The listing builds one solid part. Answer for the finished solid, in the listing's coordinates (mm). Give positions to 0.01 mm unless a question says otherwise; leave off trailing zeros. Loops run counter-clockwise (first coordinate to the right, second up) from the corner with the lowest first, then second, coordinate; pieces in that order, holes last. Notation, with made-up numbers: (-5.75, 38) - (-0.75, 38) arc R28 ccw to (-0.75, 58) - close; hole circle Ø10 at (-30.5, -27.5). An arc over 180 degrees is marked (long way). Answer as CSV lines item,"result". Start each with the question number.
1) A cutting plane is placed at A-A (x = -32.5). Determine the outline of the cut face in (y, z), and give its area (3 significant figures).
2) Flat-ended cylindrical pins translate along their axes: pin 1 (8 mm diameter, centred on x = 179, y = 432.5, fed in from +Z); pin 2 (3.5 mm diameter, centred on x = -203.2, y = 0, fed in from +Z). Find the tip coordinate at first contact, or state that the pin passes through.
3) A cutting plane is placed at C-C (z = 2). Determine the outline of the cut face in (x, y) (3 decimals), and give its area (3 significant figures).
4) A cutting plane is placed at B-B (y = -341). Determine the outline of the cut face in (x, z).
5) Find the intervals of material crossed by line 1 along Y through (x, z) = (-203.2, 5.5); line 2 along X through (y, z) = (787.4, 6.75); line 3 along X through (y, z) = (446, 3.75), in increasing order.
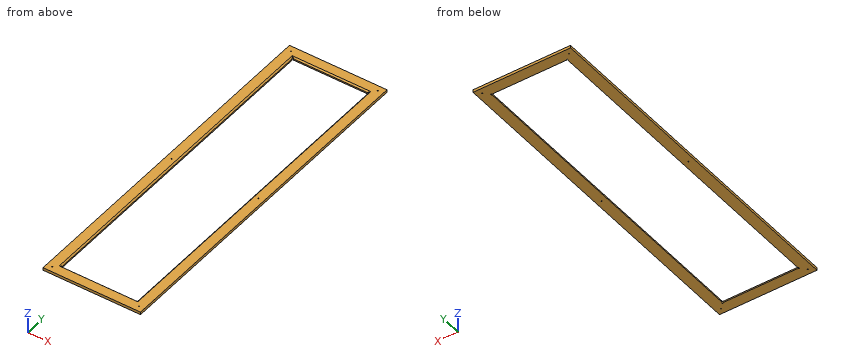
```python
from build123d import *

# Parameters (mm, degrees)
F0_W     = 457.2
F0_H     = 1625.6
F0_W_2   = 355.6
F0_H_2   = 1524
F1_DEPTH = 12.7
F2_SIZE  = 6.35
F3_R     = 3.175
F4_DEPTH = 12.7
F5_R     = 2.15265
F6_DEPTH = 12.7


with BuildPart() as f1:
    # F0 (on Top) → F1 (new body)
    with BuildSketch(Plane.XY):
        Rectangle(F0_W, F0_H)
        Rectangle(F0_W_2, F0_H_2, mode=Mode.SUBTRACT)
    extrude(amount=F1_DEPTH)

    # F2
    f2_edges = [f1.edges().sort_by_distance(p)[0] for p in [
        (0, 762, 12.7),
        (-177.8, 0, 12.7),
        (177.8, 0, 12.7),
        (0, -762, 12.7),
    ]]
    chamfer(f2_edges, length=F2_SIZE)

    # F3 (on face) → F4 (cut, through all)
    with BuildSketch(Plane(origin=(0, 0, 0), x_dir=(1, 0, 0), z_dir=(0, 0, -1))):
        with Locations((-177.8, -762)):
            Circle(F3_R)
        with Locations((177.8, -762)):
            Circle(F3_R)
        with Locations((177.8, 762)):
            Circle(F3_R)
        with Locations((-177.8, 762)):
            Circle(F3_R)
    extrude(amount=-F4_DEPTH, mode=Mode.SUBTRACT)

    # F5 (on face) → F6 (cut, through all)
    with BuildSketch(Plane.XY.offset(12.7)):
        with Locations((-203.2, -787.4)):
            Circle(F5_R)
        with Locations((203.2, -787.4)):
            Circle(F5_R)
        with Locations((203.2, 0)):
            Circle(F5_R)
        with Locations((-203.2, 0)):
            Circle(F5_R)
        with Locations((-203.2, 787.4)):
            Circle(F5_R)
        with Locations((203.2, 787.4)):
            Circle(F5_R)
    extrude(amount=-F6_DEPTH, mode=Mode.SUBTRACT)


solid = f1.part
```
Ans:
1,outline,"(-812.8, 0) - (-762, 0) - (-762, 6.35) - (-768.35, 12.7) - (-812.8, 12.7) - close; (762, 0) - (812.8, 0) - (812.8, 12.7) - (768.35, 12.7) - (762, 6.35) - close"
1,area,"1,250 mm2"
2,pin 1,"z = 11.55"
2,pin 2,"through"
3,outline,"(-228.6, -812.8) - (228.6, -812.8) - (228.6, 812.8) - (-228.6, 812.8) - close; hole circle Ø4.305 at (-203.2, -787.4); hole circle Ø4.305 at (-203.2, 0); hole circle Ø4.305 at (-203.2, 787.4); hole (-177.8, -758.825) arc R3.175 ccw (long way) to (-174.625, -762) - (174.625, -762) arc R3.175 ccw (long way) to (177.8, -758.825) - (177.8, 758.825) arc R3.175 ccw (long way) to (174.625, 762) - (-174.625, 762) arc R3.175 ccw (long way) to (-177.8, 758.825) - close; hole circle Ø4.305 at (203.2, -787.4); hole circle Ø4.305 at (203.2, 0); hole circle Ø4.305 at (203.2, 787.4)"
3,area,"201,000 mm2"
4,outline,"(-228.6, 0) - (-177.8, 0) - (-177.8, 6.35) - (-184.15, 12.7) - (-228.6, 12.7) - close; (177.8, 0) - (228.6, 0) - (228.6, 12.7) - (184.15, 12.7) - (177.8, 6.35) - close"
5,line 1,"-812.8 to -789.55, -785.25 to -2.15, 2.15 to 785.25, 789.55 to 812.8"
5,line 2,"-228.6 to -205.35, -201.05 to 201.05, 205.35 to 228.6"
5,line 3,"-228.6 to -177.8, 177.8 to 228.6"
